Part model, mm, in its own coordinate system. Face numbers are marked on the shaded views. Coordinates: 2 decimals unless noted, no trailing zeros. Write each loop counter-clockwise with the first axis right and the second up, starting at its lowest first coordinate (ties: lowest second). Pieces come first, ordered by that corner, then holes. Notation, with made-up numbers: (87.25, 63.5) - (97.25, 63.5) arc R17 ccw to (97.25, 82.5) - close; hole circle Ø7 at (41, -5.75). An arc over 180 degrees is marked (long way). Write each question's results on one line, items separated by ' | '.
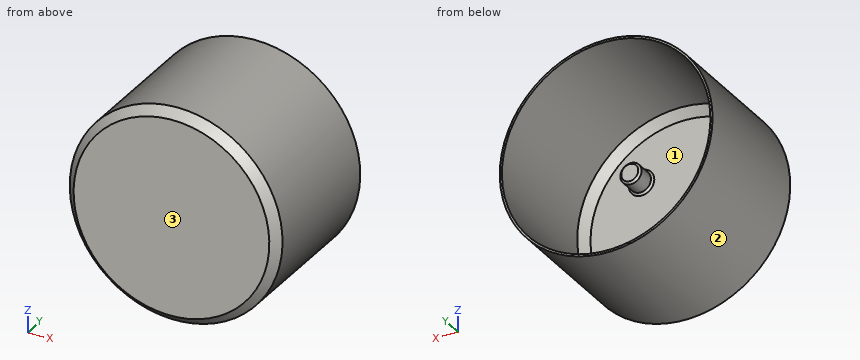
from build123d import *

# Parameters (mm, degrees)
SKETCH1_R                = 50
SKETCH1_R_2              = 49
MAIN_WALL_DEPTH          = 70
SKETCH2_R                = 50
FLOOR_2_DEPTH            = 2
INNER_FLOOR_CHAMFER_SIZE = 4
OUTER_FLOOR_CHAMFER_SIZE = 4
SKETCH3_R                = 5
CONNECTOR_PEG_DEPTH      = 10
PEG_CHAMFER_SIZE         = 1
CHAMFER1_SIZE            = 1


with BuildPart() as part:
    # Sketch1 → Main Wall (new body)
    with BuildSketch(Plane(origin=(0, 0, 0), x_dir=(1, 0, 0), z_dir=(0, 1, 0))):
        with Locations(Location((0, 0, 0), (0, 0, 270))):
            Circle(SKETCH1_R)
        with Locations(Location((0, 0, 0), (0, 0, 270))):
            Circle(SKETCH1_R_2, mode=Mode.SUBTRACT)
    extrude(amount=MAIN_WALL_DEPTH)

    # Sketch2 → Floor 2 (add)
    with BuildSketch(Plane.XZ):
        with Locations(Location((0, 0, 0), (0, 0, 90))):
            Circle(SKETCH2_R)
    extrude(amount=-FLOOR_2_DEPTH)

    # Inner Floor Chamfer
    inner_floor_chamfer_edges = [part.edges().sort_by_distance(p)[0] for p in [
        (0, 2, -49),
    ]]
    chamfer(inner_floor_chamfer_edges, length=INNER_FLOOR_CHAMFER_SIZE)

    # Outer Floor Chamfer
    outer_floor_chamfer_edges = [part.edges().sort_by_distance(p)[0] for p in [
        (0, 0, -50),
    ]]
    chamfer(outer_floor_chamfer_edges, length=OUTER_FLOOR_CHAMFER_SIZE)

    # Sketch3 → Connector Peg (add)
    with BuildSketch(Plane(origin=(0, 2, 0), x_dir=(1, 0, 0), z_dir=(0, 1, 0))):
        with Locations(Location((-21, 21, 0), (0, 0, 90))):
            Circle(SKETCH3_R)
        with Locations(Location((21, 21, 0), (0, 0, 90))):
            Circle(SKETCH3_R)
        with Locations(Location((21, -21, 0), (0, 0, 90))):
            Circle(SKETCH3_R)
        with Locations(Location((-21, -21, 0), (0, 0, 90))):
            Circle(SKETCH3_R)
    extrude(amount=CONNECTOR_PEG_DEPTH)

    # Peg Chamfer
    peg_chamfer_edges = [part.edges().sort_by_distance(p)[0] for p in [
        (-21, 12, -16),
        (21, 12, -16),
        (21, 12, 26),
        (-21, 12, 26),
    ]]
    chamfer(peg_chamfer_edges, length=PEG_CHAMFER_SIZE)

    # Chamfer1
    chamfer1_edges = [part.edges().sort_by_distance(p)[0] for p in [
        (-21, 2, -16),
        (21, 2, -16),
        (21, 2, 26),
        (-21, 2, 26),
    ]]
    chamfer(chamfer1_edges, length=CHAMFER1_SIZE)


solid = part.part
(1) Two-plate mould, pull along Z, no slides. Class the marked faces 1, 2 and 3: released by +Z, released by -Z, zero draft, split by the parting line, or undercut.
Return value:
face 1: undercut | face 2: split by the parting line | face 3: zero draft
(2) Saw through at C-C on x = 0. Write the cut outline in (y, z), then the cut area to 3 significant figures.
Return value:
outline: (0, -46) - (4, -50) - (70, -50) - (70, -49) - (6, -49) - (2, -45) - (2, 45) - (6, 49) - (70, 49) - (70, 50) - (4, 50) - (0, 46) - close | area: 336 mm^2
(3) Flat gauge pins, fed straight in: P1, Ø2, axis at x = -18.5, y = 41, coming from the -Z side; P2, Ø5, axis at x = -10, y = 25.5, coming from the +Z side; P3, Ø1, axis at y = 14, z = 29, coming from the +X side. Where does each tip first touch, or does it go through?
Return value:
P1: stops at z = -46.84 | P2: stops at z = 49.43 | P3: stops at x = 41.08
(4) Saw through at B-B on z = 0. Write the cut outline in (x, y), then the cut area to 3 significant figures.
Return value:
outline: (-50, 4) - (-46, 0) - (46, 0) - (50, 4) - (50, 70) - (49, 70) - (49, 6) - (45, 2) - (-45, 2) - (-49, 6) - (-49, 70) - (-50, 70) - close | area: 336 mm^2
(5) Wall check: line 1 (X direction, y = 35, z = 0); line 2 (Z direction, x = 1, y = 22.5); line 3 (Y direction, x = 25.5, z = 31.5). Give the ranges that are in metal, low to high. Write a range as from..to.
Return value:
line 1: x = -50..-49, 49..50 | line 2: z = -49.99..-48.99, 48.99..49.99 | line 3: y = 0..2
(6) Saw through at D-D on y = 53.5. Write the cut outline in (x, z).
Return value:
outline: circle Ø100 at (0, 0); hole circle Ø98 at (0, 0)
(7) Saw through at A-A on y = 9. Write the cut outline in (x, z), then the cut area to 3 significant figures.
Return value:
outline: circle Ø100 at (0, 0); circle Ø10 at (-21, -21); circle Ø10 at (-21, 21); circle Ø10 at (21, -21); circle Ø10 at (21, 21); hole circle Ø98 at (0, 0) | area: 625 mm^2
